Here's how the part is built. I have some questions about the finished solid (model axes, mm). A direction names the side the tool comes from. Give positions to 0.01 mm unless a question says otherwise; leave off trailing zeros. Order: outer loops, then holes, each group sorted by start corner. A loop starts at its lowest first (then second) coordinate and runs counter-clockwise, first axis right, second up. Notation, with made-up numbers: M -18,-34 L 41,-34 A14 cw 41,-20 Z; hole C -38.75,17.5 d8. An arc over 180 degrees is marked long. Use one line per item in the form item = value.
from build123d import *

# Parameters (mm, degrees)
F1_DEPTH = 45
F2_R     = 2.5
F3_DEPTH = 12


with BuildPart() as f1:
    # F0 (on Front) → F1 (new body)
    with BuildSketch(Plane.XZ):
        with BuildLine():
            Line((0, -33), (0, 0))
            Line((0, 0), (-45, 0))
            Line((-45, 0), (-45, -33))
            Line((-45, -33), (-32.901954, -33))
            Line((-32.901954, -33), (-27.5, -26.562202))
            ThreePointArc((-27.5, -26.562202), (-22.5, -11.75), (-17.5, -26.562202))
            Line((-17.5, -26.562202), (-12.098046, -33))
            Line((-12.098046, -33), (0, -33))
        make_face()
    extrude(amount=F1_DEPTH)

    # F2 (on face) → F3 (cut)
    with BuildSketch(Plane.XY):
        with Locations((-38.5, -37.5)):
            Circle(F2_R)
        with Locations((-6.5, -37.5)):
            Circle(F2_R)
        with Locations((-6.5, -7.5)):
            Circle(F2_R)
        with Locations((-38.5, -7.5)):
            Circle(F2_R)
    extrude(amount=-F3_DEPTH, mode=Mode.SUBTRACT)


solid = f1.part
Q1. I need wall thicknesses on L1, parallel to Y at x = -38.5, z = -3.25; L2, parallel to X at y = -37, z = -6; L3, parallel to X at y = -9.5, z = -3.5. Which ranges of each line are inside material? Lowest first, please.
Found:
L1 = -45 to -40, -35 to -10, -5 to 0
L2 = -45 to -40.95, -36.05 to -8.95, -4.05 to 0
L3 = -45 to -40, -37 to -8, -5 to 0
Q2. I want a section at A-A on z = -20. Write out the boundary of the cut face in (x, y), then the cut area to 3 significant figures.
Found:
outline = M -45,-45 L -30.75,-45 L -30.75,0 L -45,0 Z; M -14.25,-45 L 0,-45 L 0,0 L -14.25,0 Z
area = 1,280 mm²
Q3. Thinking about a two-plate mould opening in X: for faces 1 (the face through (-7.04, -39.94, -5.92)), 2 (the face through (-45, -22, -16)), 3 (the face through (-39, -22, -33)), which applies, +X half, -X half, draft (parallel to the pull), parting line (faces both ways), or undercut?
Found:
face_1 = undercut
face_2 = -X half
face_3 = draft
Q4. I'm going to push flat-ended pins straight in: pin 1 Ø2.5 at (x, y) = (-38.5, -8.5) entering from +Z; pin 2 Ø6 at (x, y) = (-29.5, -40) entering from -Z; pin 3 Ø5 at (x, y) = (-24.5, -27.5) entering from -Z. Where does each tip first touch, or does it pass through?
Found:
pin_1 = -12
pin_2 = -32.52
pin_3 = -13.09
Q5. I want a section at D-D on z = -4.5. Write out the boundary of the cut face in (x, y).
Found:
outline = M -45,-45 L 0,-45 L 0,0 L -45,0 Z; hole C -38.5,-37.5 d5; hole C -38.5,-7.5 d5; hole C -6.5,-37.5 d5; hole C -6.5,-7.5 d5
Q6. On a 3-axis mill with a long thin cutter (end or side, diameter ignored), from which of +Z, -Z, +X, -X, +Y, -Y can I reach the whole of each face in a straight line? I mean faces 4 (the face through (-7, -7, -12)), 5 (the face through (-30.24, -22.18, -29.83)), 6 (the face through (-22, -22, 0)). Say none if no direction works.
Found:
face_4 = +Z
face_5 = -Z, +Y, -Y
face_6 = +Z, +X, -X, +Y, -Y
Q7. I want a section at B-B on y = -7.5. Write out the boundary of the cut face in (x, z).
Found:
outline = M -45,-33 L -32.9,-33 L -27.5,-26.56 A8.25 cw long -17.5,-26.56 L -12.1,-33 L 0,-33 L 0,0 L -4,0 L -4,-12 L -9,-12 L -9,0 L -36,0 L -36,-12 L -41,-12 L -41,0 L -45,0 Z
Q8. I want a section at C-C on x = -6.5. Write out the boundary of the cut face in (y, z).
Found:
outline = M -45,-33 L 0,-33 L 0,0 L -5,0 L -5,-12 L -10,-12 L -10,0 L -35,0 L -35,-12 L -40,-12 L -40,0 L -45,0 Z
